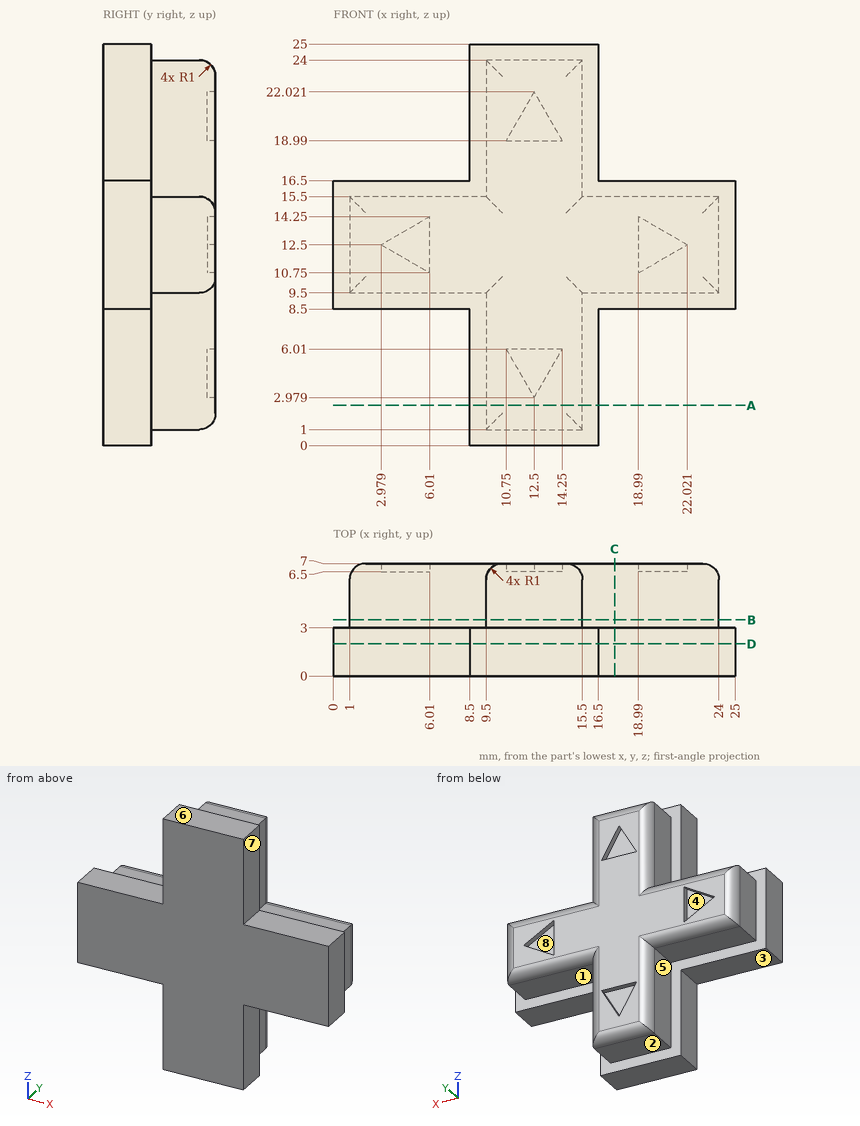
Here's the drawing with two shaded views (mm, measured from the low corner). I have some questions. A direction names the side the tool comes from. Give positions to 0.01 mm unless a question says otherwise; leave off trailing zeros. Order: outer loops, then holes, each group sorted by start corner. A loop starts at its lowest first (then second) coordinate and runs counter-clockwise, first axis right, second up.
Q1. I'm going to push flat-ended pins straight in: P1, Ø1.5, axis at x = 19, y = 4, coming from the -Z side; P2, Ø1.5, axis at x = 4.5, y = 2, coming from the -Z side; P3, Ø1.5, axis at y = 4.5, z = 13.5, coming from the +X side. Where does each tip first touch, or does it pass through?
Q2. Suppose I cut it at B-B, the plane y = 3.5. Write out the boundary of the cut face in (x, z).
Q3. We'd pull the mould along X, two halves only. Please class the marked faces 5, 6, 7 and 8: +X half, -X half, draft (parallel to the pull), parting line (faces both ways), or undercut.
Q4. Suppose I cut it at A-A, the plane z = 2.5. Write out the boundary of the cut face in (x, y).
Q5. Suppose I cut it at D-D, the plane y = 2. Write out the boundary of the cut face in (x, z), and give its area (3 significant figures).
Q6. Suppose I cut it at C-C, the plane x = 17.5. Write out the boundary of the cut face in (y, z).
Q7. For the marked faces 1, 2, 3 and 4, which set-ups out of +Z, -Z, +X, -X, +Y, -Y let a thin tool reach every point of the face, with its end or its side?
Q8. If I drill on line 1 along X through (y, z) = (6.75, 13.25) (1 decimal); line 2 along Z through (x, y) = (3.75, 5); line 3 along Z through (x, y) = (4.25, 2.75), over which ranges is the centre line in solid material (lowest first)?
Solution:
1. P1: stops at z = 9.5
1. P2: stops at z = 8.5
1. P3: stops at x = 24
2. outline: (1, 9.5) - (9.5, 9.5) - (9.5, 1) - (15.5, 1) - (15.5, 9.5) - (24, 9.5) - (24, 15.5) - (15.5, 15.5) - (15.5, 24) - (9.5, 24) - (9.5, 15.5) - (1, 15.5) - close
3. face 5: -X half
3. face 6: draft
3. face 7: +X half
3. face 8: undercut
4. outline: (8.5, 0) - (16.5, 0) - (16.5, 3) - (15.5, 3) - (15.5, 6) arc R1 ccw to (14.5, 7) - (10.5, 7) arc R1 ccw to (9.5, 6) - (9.5, 3) - (8.5, 3) - close
5. outline: (0, 8.5) - (8.5, 8.5) - (8.5, 0) - (16.5, 0) - (16.5, 8.5) - (25, 8.5) - (25, 16.5) - (16.5, 16.5) - (16.5, 25) - (8.5, 25) - (8.5, 16.5) - (0, 16.5) - close
5. area: 336 mm2
6. outline: (0, 8.5) - (3, 8.5) - (3, 9.5) - (6, 9.5) arc R1 ccw to (7, 10.5) - (7, 14.5) arc R1 ccw to (6, 15.5) - (3, 15.5) - (3, 16.5) - (0, 16.5) - close
7. face 1: -Z, +X, +Y
7. face 2: -Z, +X, -X, +Y
7. face 3: -Z, -X, +Y, -Y
7. face 4: +Y
8. line 1: x = 1.3 to 4.3, 6 to 19, 20.7 to 23.7
8. line 2: z = 9.5 to 15.5
8. line 3: z = 8.5 to 16.5
